For this review, take the finished solid that the model builds, in its own axes (mm). Face numbers are marked on the shaded views. A direction names the side the tool comes from. Coordinates: 2 decimals unless noted, no trailing zeros. One line per item, written item: value. Start each with the question number.
(1) Clearance check with flat-ended pins moving along their axes: pin 1 (0.5 mm diameter, centred on y = -33.5, z = -4.5, fed in from +X); pin 2 (11 mm diameter, centred on x = -142.78, y = -23.62, fed in from -Z); pin 3 (1.5 mm diameter, centred on x = -132.5, y = -23, fed in from -Z); pin 4 (3 mm diameter, centred on y = -27.5, z = -16.5, fed in from -X). State where each tip first meets the part, or that it passes through.
(2) To check wall thickness, follow line 1 along Z through (x, y) = (-149, -26.25); line 2 along Z through (x, y) = (-132.5, -23); line 3 along Y through (x, z) = (-145, 61). State the ranges of each line that lie inside material, in increasing order.
(3) Mouldability with a two-part tool opening along Z and no side actions: class the marked faces 4, 5, 6 and 7 as released by +Z, released by -Z, zero draft, split by the parting line, or undercut.
(4) For the marked faces 1, 2 and 3, list the 3-axis set-ups (+Z, -Z, +X, -X, +Y, -Y) from which the entire face can be reached by the end or side of a thin tool; tool diameter is ignored.
```python
from build123d import *

# Parameters (mm, degrees)
SKETCH1_R           = 6.9
SKETCH1_R_2         = 2.6
BOSS_EXTRUDE1_DEPTH = 10
BOSS_EXTRUDE2_DEPTH = 12
SKETCH3_R           = 7
SKETCH3_R_2         = 4
BOSS_EXTRUDE3_DEPTH = 4
BOSS_EXTRUDE4_DEPTH = 84
BOSS_EXTRUDE5_DEPTH = 84
CUT_EXTRUDE1_DEPTH  = 190.323263107


with BuildPart() as part:
    # Sketch1 → Boss-Extrude1 (new body)
    with BuildSketch(Plane.XY):
        with BuildLine():
            Line((-155.070766667, -34.03543395), (-139.182010536, -34.03543395))
            Line((-139.182010536, -34.03543395), (-124.735717634, -34.03543395))
            add(Edge.make_bspline(
                [(-124.735717634, -34.03543395), (-120.868070652, -30.634901056), (-118.110731489, -25.337058748)],
                knots=[0.604913823, 0.604913823, 0.604913823, 1, 1, 1], degree=2))
            ThreePointArc((-118.110731489, -25.337058748), (-114.956411592, -18.057608365), (-121.224300514, -13.194101363))
            Line((-121.224300514, -13.194101363), (-122.374915538, -13.297224598))
            Line((-122.374915538, -13.297224598), (-145.504342678, -15.370186717))
            add(Edge.make_bspline(
                [(-145.504342678, -15.370186717), (-147.665446471, -15.751951197), (-150.237941893, -16.278752791)],
                knots=[0, 0, 0, 0.143499102, 0.143499102, 0.143499102], degree=2))
            add(Edge.make_bspline(
                [(-150.237941893, -16.278752791), (-156.331446907, -19.412430802), (-156.587305002, -28.504886835), (-155.070766667, -34.03543395)],
                knots=[0, 0, 0, 0, 1, 1, 1, 1], degree=3))
        make_face()
        with Locations((-142.777717077, -23.619181221)):
            Circle(SKETCH1_R, mode=Mode.SUBTRACT)
        with Locations((-121.224300514, -19.664754316)):
            Circle(SKETCH1_R_2, mode=Mode.SUBTRACT)
    boss_extrude1 = extrude(amount=BOSS_EXTRUDE1_DEPTH)

    # Sketch2 → Boss-Extrude2 (add)
    with BuildSketch(Plane(origin=(0, 0, 0), x_dir=(-1, 0, 0), z_dir=(0, 0, -1))):
        with BuildLine():
            Line((124.810828249, -34.03543395), (124.810828249, -33.03543395))
            ThreePointArc((124.810828249, -33.03543395), (125.396614687, -31.621220388), (126.810828249, -31.03543395))
            Line((126.810828249, -31.03543395), (155.660238601, -31.03543395))
            add(Edge.make_bspline(
                [(155.660238601, -31.03543395), (155.453340821, -32.220849379), (155.070766667, -34.03543395)],
                knots=[0.469279702, 0.469279702, 0.469279702, 1.113861257, 1.113861257, 1.113861257], degree=2))
            Line((155.070766667, -34.03543395), (124.810828249, -34.03543395))
        make_face()
    extrude(amount=BOSS_EXTRUDE2_DEPTH)

    # Mirror1: Boss-Extrude1 across plane
    add(boss_extrude1.mirror(Plane(origin=(0, 0, -6), x_dir=(1, 0, 0), z_dir=(0, 0, -1))))

    # Sketch3 → Boss-Extrude3 (add)
    with BuildSketch(Plane(origin=(0, 0, 0), x_dir=(-1, 0, 0), z_dir=(0, 0, -1))):
        with Locations((142.777717077, -23.619181221)):
            Circle(SKETCH3_R)
        with Locations((142.777717077, -23.619181221)):
            Circle(SKETCH3_R_2, mode=Mode.SUBTRACT)
    boss_extrude3 = extrude(amount=-BOSS_EXTRUDE3_DEPTH)

    # Mirror2: Boss-Extrude3 across plane
    add(boss_extrude3.mirror(Plane(origin=(0, 0, -6), x_dir=(1, 0, 0), z_dir=(0, 0, -1))))

    # Sketch4 → Boss-Extrude4 (add)
    with BuildSketch(Plane.XY.offset(10)):
        with BuildLine():
            add(Edge.make_bspline(
                [(-155.660238601, -31.03543395), (-155.52477055, -32.104378324), (-155.322110933, -33.11882586), (-155.070766667, -34.03543395)],
                knots=[0.834264482, 0.834264482, 0.834264482, 0.834264482, 1, 1, 1, 1], degree=3))
            Line((-155.070766667, -34.03543395), (-124.735717634, -34.03543395))
            add(Edge.make_bspline(
                [(-124.735717634, -34.03543395), (-123.199822379, -32.685036057), (-121.8390218, -31.03543395)],
                knots=[0, 0, 0, 1, 1, 1], degree=2))
            Line((-121.8390218, -31.03543395), (-155.660238601, -31.03543395))
        make_face()
    extrude(amount=BOSS_EXTRUDE4_DEPTH)

    # Sketch5 → Boss-Extrude5 (add)
    with BuildSketch(Plane(origin=(0, 0, -22), x_dir=(-1, 0, 0), z_dir=(0, 0, -1))):
        with BuildLine():
            Line((155.070766667, -34.03543395), (124.735717633, -34.035433949))
            add(Edge.make_bspline(
                [(124.735717633, -34.035433949), (123.199822378, -32.685036056), (121.8390218, -31.03543395)],
                knots=[0, 0, 0, 1, 1, 1], degree=2))
            Line((121.8390218, -31.03543395), (155.660238601, -31.03543395))
            add(Edge.make_bspline(
                [(155.660238601, -31.03543395), (155.52477055, -32.104378324), (155.322110933, -33.11882586), (155.070766667, -34.03543395)],
                knots=[0.834264482, 0.834264482, 0.834264482, 0.834264482, 1, 1, 1, 1], degree=3))
        make_face()
    extrude(amount=BOSS_EXTRUDE5_DEPTH)

    # Sketch6 → Cut-Extrude1 (cut, through all)
    with BuildSketch(Plane(origin=(0, -31.03543395, 0), x_dir=(1, 0, 0), z_dir=(0, 1, 0))):
        Polygon((-137.786415389, 76.894835229), (-142.400005748, 77.114191864), (-144.516832509, 81.219356636), (-142.02006891, 85.105164771), (-137.406478551, 84.885808136), (-135.289651791, 80.780643364), align=None)
        Polygon((-135.289651791, 30.780643364), (-137.786415389, 26.894835229), (-142.400005748, 27.114191864), (-144.516832509, 31.219356636), (-142.02006891, 35.105164771), (-137.406478551, 34.885808136), align=None)
        with BuildLine():
            Line((-155.6602386, 22), (-173.465321409, 22))
            Line((-173.465321409, 22), (-173.465321409, 117.834139367))
            Line((-173.465321409, 117.834139367), (-100.430925903, 117.834139367))
            Line((-100.430925903, 117.834139367), (-121.8390218, 22))
            add(Edge.make_bspline(
                [(-121.8390218, 22), (-130.237957541, 29.288236007), (-131.708688401, 51.819501052), (-127.475857655, 72.230953717), (-131.071963897, 82.863468574)],
                knots=[0, 0, 0, 0, 0.490729359, 1, 1, 1, 1], degree=3))
            ThreePointArc((-131.071963897, 82.863468574), (-140.840035974, 89.976993263), (-148.928982602, 81))
            add(Edge.make_bspline(
                [(-148.928982602, 81), (-152.625386512, 74.081760345), (-155.262352814, 54.105117148), (-154.402874629, 34.24459948), (-155.6602386, 22)],
                knots=[0, 0, 0, 0, 0.385424941, 1, 1, 1, 1], degree=3))
        make_face()
        with BuildLine():
            Line((-100.430925903, -105.834139367), (-121.8390218, -10))
            add(Edge.make_bspline(
                [(-121.8390218, -10), (-130.237957541, -17.288236007), (-131.708688401, -39.819501052), (-127.475857655, -60.230953717), (-131.071963897, -70.863468574)],
                knots=[0, 0, 0, 0, 0.490729359, 1, 1, 1, 1], degree=3))
            ThreePointArc((-131.071963897, -70.863468574), (-140.840035974, -77.976993263), (-148.928982602, -69))
            add(Edge.make_bspline(
                [(-148.928982602, -69), (-152.625386512, -62.081760345), (-155.262352814, -42.105117148), (-154.402874629, -22.24459948), (-155.6602386, -10)],
                knots=[0, 0, 0, 0, 0.385424941, 1, 1, 1, 1], degree=3))
            Line((-155.6602386, -10), (-173.465321409, -10))
            Line((-173.465321409, -10), (-173.465321409, -105.834139367))
            Line((-173.465321409, -105.834139367), (-100.430925903, -105.834139367))
        make_face()
        Polygon((-142.02006891, -23.105164771), (-137.406478551, -22.885808136), (-135.289651791, -18.780643364), (-137.786415389, -14.894835229), (-142.400005748, -15.114191864), (-144.516832509, -19.219356636), align=None)
        Polygon((-135.289651791, -68.780643364), (-137.786415389, -64.894835229), (-142.400005748, -65.114191864), (-144.516832509, -69.219356636), (-142.02006891, -73.105164771), (-137.406478551, -72.885808136), align=None)
    extrude(amount=-CUT_EXTRUDE1_DEPTH, mode=Mode.SUBTRACT)


solid = part.part
```
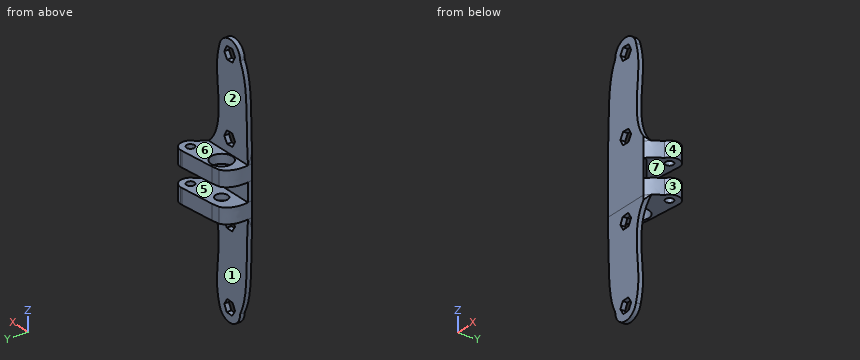
Geometry check:
1. pin 1: stops at x = -124.81
1. pin 2: stops at z = -16
1. pin 3: stops at z = -22
1. pin 4: stops at x = -155.85
2. line 1: z = -16 to -12, 0 to 4
2. line 2: z = -22 to -12, 0 to 10
2. line 3: y = -34.04 to -31.04
3. face 4: zero draft
3. face 5: undercut
3. face 6: released by +Z
3. face 7: undercut
4. face 1: -Z, +X, -X, +Y
4. face 2: +Z, +X, -X, +Y
4. face 3: +Z, -Z, +X
